Can you work these out from the model? Positions are in its coordinate system, mm. Give positions to 0.01 mm unless a question says otherwise; leave off trailing zeros. Write each loop counter-clockwise with the first axis right and the second up, starting at its lowest first coordinate (ties: lowest second). Pieces come first, ordered by that corner, then holes. Notation, with made-up numbers: (-4.5, 79.25) - (9.5, 79.25) arc R5 ccw to (9.5, 87.25) - close; hole circle Ø5 at (50, -4.5). An arc over 180 degrees is marked (long way). Return JSON: item names as keys, results as strings. Group by question number.
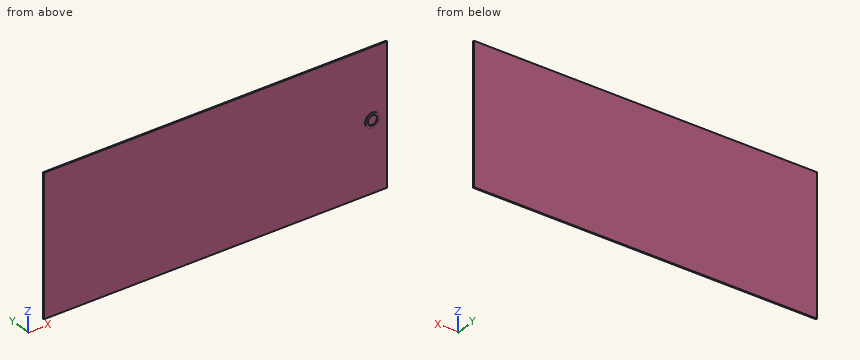
from build123d import *

# Parameters (mm, degrees)
F0_W     = 895.35
F0_H     = 365.252
F1_DEPTH = 3.175
F2_R     = 19.05
F2_R_2   = 12.7
F3_DEPTH = 1.524
F4_DEPTH = 1.524


with BuildPart() as f1:
    # F0 (on Front) → F1 (new body)
    with BuildSketch(Plane.XZ):
        Rectangle(F0_W, F0_H)
    extrude(amount=F1_DEPTH)

    # F2 (on face) → F3 (join)
    with BuildSketch(Plane.XZ.offset(3.175)):
        with Locations((409.575, 0)):
            Circle(F2_R)
        with Locations((409.575, 0)):
            Circle(F2_R_2, mode=Mode.SUBTRACT)
    extrude(amount=F3_DEPTH)

    # F4 (cut): a face of the model
    f4_faces = [f1.faces().sort_by_distance(p)[0] for p in [
        (409.575, -3.175, 0),
    ]]
    extrude(f4_faces, amount=-F4_DEPTH, mode=Mode.SUBTRACT)


solid = f1.part
1) Imagine slicing it at B-B, the plane x = -384.5. Write out the boundary of the cut face in (y, z) (3 decimals), and give its area (3 significant figures).
2) Imagine slicing it at C-C, the plane z = -56. Write out the boundary of the cut face in (x, y) (3 decimals).
3) Imagine slicing it at A-A, the plane z = 0. Write out the boundary of the cut face in (x, y) (3 decimals).
4) Will this pin go through, and if not, where does the flat tip stop? pin 1 Ø12.5 at (x, z) = (406.5, 3.5) entering from -Y.
5) I need wall thicknesses on line 1 along Y through (x, z) = (125.5, 123) (3 decimals); line 2 along X through (y, z) = (-3, -3.5) (3 decimals). Which ranges of each line are inside material? Lowest first, please.
Resolved:
{
 "1": {"outline": "(-3.175, -182.626) - (0, -182.626) - (0, 182.626) - (-3.175, 182.626) - close", "area": "1,160 mm^2"},
 "2": {"outline": "(-447.675, -3.175) - (447.675, -3.175) - (447.675, 0) - (-447.675, 0) - close"},
 "3": {"outline": "(-447.675, -3.175) - (390.525, -3.175) - (390.525, -4.699) - (396.875, -4.699) - (396.875, -1.651) - (422.275, -1.651) - (422.275, -4.699) - (428.625, -4.699) - (428.625, -3.175) - (447.675, -3.175) - (447.675, 0) - (-447.675, 0) - close"},
 "4": {"pin 1": "y = -1.65"},
 "5": {"line 1": "-3.175 to 0", "line 2": "-447.675 to 397.367, 421.783 to 447.675"}
}
